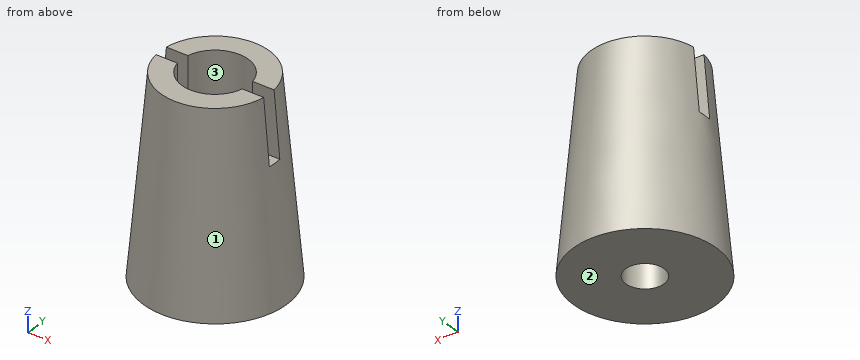
```python
from build123d import *

# Parameters (mm, degrees)
F2_R     = 10.625
F0_R     = 14
F4_R     = 3.75
F5_DEPTH = 61.90218
F7_DEPTH = 12.5
F9_D     = 13
F9_DEPTH = 8.5
F9_TIP   = 3.9055940237


with BuildPart() as f3:
    # F2 (on offset) → F3 section 0
    with BuildSketch(Plane.XY.offset(38)):
        Circle(F2_R)
    # F0 (on Top) → F3 section 1
    with BuildSketch(Plane.XY):
        Circle(F0_R)
    loft()

    # F4 (on Top) → F5 (cut)
    with BuildSketch(Plane.XY):
        Circle(F4_R)
    extrude(amount=F5_DEPTH, mode=Mode.SUBTRACT)

    # F6 (on face) → F7 (cut)
    with BuildSketch(Plane.XY.offset(38)):
        with BuildLine():
            Line((-10.5356537529, 1.375), (-16.0871957117, 1.375))
            Line((-16.0871957117, 1.375), (-16.0871957117, 0))
            Line((-16.0871957117, 0), (-10.625, 0))
            ThreePointArc((-10.625, 0), (-10.60263991, 0.6889498806), (-10.5356537529, 1.375))
        make_face()
        with BuildLine():
            Line((-3.4888214342, 1.375), (-10.5356537529, 1.375))
            ThreePointArc((-10.5356537529, 1.375), (-10.60263991, 0.6889498806), (-10.625, 0))
            Line((-10.625, 0), (-3.75, 0))
            ThreePointArc((-3.75, 0), (-3.6841267879, 0.6997926913), (-3.4888214342, 1.375))
        make_face()
        with BuildLine():
            Line((-10.625, 0), (-16.0871957117, 0))
            Line((-16.0871957117, 0), (-16.0871957117, -1.375))
            Line((-16.0871957117, -1.375), (-10.5356537529, -1.375))
            ThreePointArc((-10.5356537529, -1.375), (-10.60263991, -0.6889498806), (-10.625, 0))
        make_face()
        with BuildLine():
            ThreePointArc((10.625, 0), (10.60263991, 0.6889498806), (10.5356537529, 1.375))
            Line((10.5356537529, 1.375), (3.4888214342, 1.375))
            ThreePointArc((3.4888214342, 1.375), (3.6841267879, 0.6997926913), (3.75, 0))
            Line((3.75, 0), (10.625, 0))
        make_face()
        with BuildLine():
            Line((16.6521480927, 1.375), (10.5356537529, 1.375))
            ThreePointArc((10.5356537529, 1.375), (10.60263991, 0.6889498806), (10.625, 0))
            Line((10.625, 0), (16.6521480927, 0))
            Line((16.6521480927, 0), (16.6521480927, 1.375))
        make_face()
        with BuildLine():
            Line((-3.75, 0), (-10.625, 0))
            ThreePointArc((-10.625, 0), (-10.60263991, -0.6889498806), (-10.5356537529, -1.375))
            Line((-10.5356537529, -1.375), (-3.4888214342, -1.375))
            ThreePointArc((-3.4888214342, -1.375), (-3.6841267879, -0.6997926913), (-3.75, 0))
        make_face()
        with BuildLine():
            ThreePointArc((10.5356537529, -1.375), (10.60263991, -0.6889498806), (10.625, 0))
            Line((10.625, 0), (3.75, 0))
            ThreePointArc((3.75, 0), (3.6841267879, -0.6997926913), (3.4888214342, -1.375))
            Line((3.4888214342, -1.375), (10.5356537529, -1.375))
        make_face()
        with BuildLine():
            Line((16.6521480927, 0), (10.625, 0))
            ThreePointArc((10.625, 0), (10.60263991, -0.6889498806), (10.5356537529, -1.375))
            Line((10.5356537529, -1.375), (16.6521480927, -1.375))
            Line((16.6521480927, -1.375), (16.6521480927, 0))
        make_face()
    extrude(amount=-F7_DEPTH, mode=Mode.SUBTRACT)

    # F9
    with Locations(Plane.XY.offset(38)):
        with Locations((0, 0)):
            Hole(F9_D / 2, depth=F9_DEPTH)
            with Locations((0, 0, -(F9_DEPTH + F9_TIP / 2))):  # 118° drill point
                Cone(0, F9_D / 2, F9_TIP, mode=Mode.SUBTRACT)


solid = f3.part
```
Could you check a few things on this model? Use its own coordinates, in mm. Face numbers are marked on the shaded views. Round coordinates to 2 decimals unless told otherwise and drop trailing zeros. Order: outer loops, then holes, each group sorted by start corner. A loop starts at its lowest first (then second) coordinate and runs counter-clockwise, first axis right, second up. Notation, with made-up numbers: M -12,86 L -3,86 A13 cw -3,96 Z; hole C 60,44.5 d7. An arc over 180 degrees is marked long. One line per question, with ' | ' between items. Start each with the question number.
(1) Thinking about a two-plate mould opening in Y: for the marked faces 1, 2 and 3, which applies, +Y half, -Y half, draft (parallel to the pull), parting line (faces both ways), or undercut?
(2) Suppose I cut it at D-D on z = 26. List the corners of the cut face in (x, y) for me (3 decimals).
(3) Suppose I cut it at B-B on z = 33.5. List the corners of the cut face in (x, y) for me (3 decimals), then the cut area to 3 significant figures.
(4) Please list where these lines run through material, in increasing order: line 1 along Y through (x, z) = (3.5, 35); line 2 along Y through (x, z) = (0, 11.75); line 3 along X through (y, z) = (0, 9.25).
(5) Suppose I cut it at A-A on x = 0. List the corners of the cut face in (y, z) for me (3 decimals), then the cut area to 3 significant figures.
(6) Suppose I cut it at C-C on z = 15. List the corners of the cut face in (x, y) for me, then the cut area to 3 significant figures.
(7) For P1, Ø2.5, axis at x = 7, z = 32, coming from the -Y side; P2, Ø4, axis at x = -1.5, z = 14.5, coming from the -Y side; P3, Ø3, axis at y = 3, z = 33.5, coming from the +X side, each with a flat end and sliding along its axis, tell me the tip position at first contact or that it passes through.
Geometry results:
1) face 1: parting line | face 2: draft | face 3: undercut
2) outline: M -11.61,-1.375 A11.691 ccw 11.61,-1.375 L 3.489,-1.375 A3.75 cw -3.489,-1.375 Z; M -11.61,1.375 L -3.489,1.375 A3.75 cw 3.489,1.375 L 11.61,1.375 A11.691 ccw Z
3) outline: M -10.939,-1.375 A11.025 ccw 10.939,-1.375 L 6.353,-1.375 A6.5 cw -6.353,-1.375 Z; M -10.939,1.375 L -6.353,1.375 A6.5 cw 6.353,1.375 L 10.939,1.375 A11.025 ccw Z | area: 224 mm²
4) line 1: -10.31 to -5.48, 5.48 to 10.31 | line 2: -12.96 to -3.75, 3.75 to 12.96 | line 3: -13.18 to -3.75, 3.75 to 13.18
5) outline: M -14,0 L -3.75,0 L -3.75,27.848 L -6.5,29.5 L -6.5,38 L -10.625,38 Z; M 3.75,0 L 14,0 L 10.625,38 L 6.5,38 L 6.5,29.5 L 3.75,27.848 Z | area: 599 mm²
6) outline: C 0,0 d25.34; hole C 0,0 d7.5 | area: 460 mm²
7) P1: y = -9.57 | P2: y = -12.86 | P3: x = 10.96
